```python
from build123d import *

# Parameters (mm, degrees)
SKETCH1_W           = 100
SKETCH1_H           = 100
SKETCH1_W_2         = 87
SKETCH1_H_2         = 87
BOSS_EXTRUDE1_DEPTH = 2.5
BOSS_EXTRUDE2_DEPTH = 2.5
SKETCH3_W           = 52.284767499
SKETCH3_H           = 7.135478262
CUT_EXTRUDE1_DEPTH  = 2.5
SKETCH4_R           = 3
CUT_EXTRUDE2_DEPTH  = 2.5
EXTRUDE_THIN2_DEPTH = 2.5
SKETCH6_R           = 5.5
BOSS_EXTRUDE3_DEPTH = 2.5


with BuildPart() as part:
    # Sketch1 → Boss-Extrude1 (new body)
    with BuildSketch(Plane(origin=(0, 0, 0), x_dir=(1, 0, 0), z_dir=(0, 1, 0))):
        Rectangle(SKETCH1_W, SKETCH1_H)
        Rectangle(SKETCH1_W_2, SKETCH1_H_2, mode=Mode.SUBTRACT)
    extrude(amount=BOSS_EXTRUDE1_DEPTH)

    # Sketch2 → Boss-Extrude2 (add)
    with BuildSketch(Plane(origin=(0, 2.5, 0), x_dir=(1, 0, 0), z_dir=(0, 1, 0))):
        with BuildLine():
            Line((-12.615137118, -35.5), (12.615137118, -35.5))
            ThreePointArc((12.615137118, -35.5), (20.615137118, -43.5), (12.615137118, -51.5))
            Line((12.615137118, -51.5), (-12.615137118, -51.5))
            ThreePointArc((-12.615137118, -51.5), (-20.615137118, -43.5), (-12.615137118, -35.5))
        make_face()
    extrude(amount=-BOSS_EXTRUDE2_DEPTH)

    # Sketch3 → Cut-Extrude1 (cut)
    with BuildSketch(Plane(origin=(0, 2.5, 0), x_dir=(1, 0, 0), z_dir=(0, 1, 0))):
        with Locations((-0.902498863, -53.567739131)):
            Rectangle(SKETCH3_W, SKETCH3_H)
    extrude(amount=-CUT_EXTRUDE1_DEPTH, mode=Mode.SUBTRACT)

    # Sketch4 → Cut-Extrude2 (cut)
    with BuildSketch(Plane(origin=(0, 2.5, 0), x_dir=(1, 0, 0), z_dir=(0, 1, 0))):
        with Locations(Location((-0.710916126, -40.5, 0), (0, 0, 270))):
            Circle(SKETCH4_R)
    extrude(amount=-CUT_EXTRUDE2_DEPTH, mode=Mode.SUBTRACT)

    # Sketch5 → Extrude-Thin2 (add)
    with BuildSketch(Plane(origin=(0, 2.5, 0), x_dir=(1, 0, 0), z_dir=(0, 1, 0))):
        Polygon((-42.268876098, -45.959031097), (48.231095848, -0.649852738), (45.768848044, 4.268209457), (-44.731123902, -41.040968903), align=None)
        Polygon((44.727203432, -41.039010009), (-46.134206752, 4.270168351), (-48.588613617, -0.651811631), (42.272796568, -45.960989991), align=None)
    extrude(amount=-EXTRUDE_THIN2_DEPTH)

    # Sketch6 → Boss-Extrude3 (add)
    with BuildSketch(Plane(origin=(0, 2.5, 0), x_dir=(1, 0, 0), z_dir=(0, 1, 0))):
        with Locations((37.337615019, -43.5)):
            Circle(SKETCH6_R)
        with Locations((43.5, -3.018495081)):
            Circle(SKETCH6_R)
        with Locations((-37.337615019, -43.5)):
            Circle(SKETCH6_R)
        with Locations((-43.5, -3.018495081)):
            Circle(SKETCH6_R)
    extrude(amount=-BOSS_EXTRUDE3_DEPTH)


solid = part.part
```
Work out the finished part from the listing and answer in its coordinate system (mm). A direction names the side the tool comes from. Coordinates: 2 decimals unless noted, no trailing zeros. Loops run counter-clockwise (first coordinate to the right, second up) from the corner with the lowest first, then second, coordinate; pieces in that order, holes last.
1) Section C-C (y = 2.1) is taken. Give the number of separate pieces and of enclosed holes in the cut face, plus the area to 3 significant figures.
Results:
separate pieces: 1
enclosed holes: 5
area: 3,770 mm2
2) Consider probe 1 along Z at (x, y) = (18, 2); probe 2 along Z at (x, y) = (-27, 0.9); probe 3 along X at (y, z) = (0.75, 40.5). Determine where each line is inside the solid, lowest interval first.
Results:
probe 1: z = -50 to -43.5, 9.63 to 15.79, 27.71 to 33.86, 37.58 to 50
probe 2: z = -50 to -43.5, 5.27 to 11.42, 32.16 to 38.31, 43.5 to 50
probe 3: x = -50 to -31.37, -20.03 to -3.71, 2.29 to 20.03, 31.32 to 50
3) Section B-B (z = 26.5) is taken. Give the vertices of the cut face in (x, y).
Results:
outline: (-50, 0) - (-43.5, 0) - (-43.5, 2.5) - (-50, 2.5) - close; (-15.69, 0) - (-3.4, 0) - (-3.4, 2.5) - (-15.69, 2.5) - close; (3.25, 0) - (15.57, 0) - (15.57, 2.5) - (3.25, 2.5) - close; (43.5, 0) - (50, 0) - (50, 2.5) - (43.5, 2.5) - close
4) Section A-A (z = -33.5) is taken. Give the vertices of the cut face in (x, y).
Results:
outline: (-50, 0) - (-43.5, 0) - (-43.5, 2.5) - (-50, 2.5) - close; (43.5, 0) - (50, 0) - (50, 2.5) - (43.5, 2.5) - close
5) For faces 4 (the flat face through (-43.5, 1, -23)), 5 (the flat face through (-1, 0, 22)), determine the directions among +Z, -Z, +X, -X, +Y, -Y from which every point of the face is accessible in a straight line to the end or side of a thin tool.
Results:
face 4: +Y, -Y
face 5: +Z, -Z, +X, -X, -Y
6) For a pull along X with two mould halves and no side action, classify faces 1 (the cylindrical face through (31.99, 1.27, 42.22)), 2 (the flat face through (-1, 1, -50)), 3 (the flat face through (50, 1, 1)) as +X half, -X half, draft (parallel to the pull), parting line (faces both ways), or undercut.
Results:
face 1: undercut
face 2: draft
face 3: +X half
7) Section D-D (z = 3.5) is taken. Give the vertices of the cut face in (x, y), plus the area to 3 significant figures.
Results:
outline: (-50, 0) - (-30.55, 0) - (-30.55, 2.5) - (-50, 2.5) - close; (30.25, 0) - (50, 0) - (50, 2.5) - (30.25, 2.5) - close
area: 98.0 mm2
